Verification items for the finished model (mm, model axes). Round coordinates to 2 decimals unless told otherwise and drop trailing zeros. Order: outer loops, then holes, each group sorted by start corner. A loop starts at its lowest first (then second) coordinate and runs counter-clockwise, first axis right, second up. Notation, with made-up numbers: (-32, 82) -> (-8, 82) arc R21 ccw to (-8, 88) -> close; hole circle Ø4 at (-20, -27.75). An arc over 180 degrees is marked (long way). Put each result on its own line as item: value.
from build123d import *

# Parameters (mm, degrees)
CLAMP_AND_LOWER_FOOT_DEPTH = 14
SKETCH_2_R                 = 57.15
CANISTER_SEAT_DEPTH        = 89.959640287


with BuildPart() as part:
    # 草图1 → Clamp_and_lower_foot (new body)
    with BuildSketch(Plane.XY):
        Polygon((39.852831801, -47.494755473), (43.840620434, -43.840620434), (47.494755473, -39.852831801), (50.787426746, -35.561739054), (53.693575035, -31), (56.191082796, -26.202332228), (58.260942489, -21.205248886), (59.88740123, -16.046780796), (61.058080687, -10.766187015), (61.764071282, -5.40365605), (62, 0), (61.764071282, 5.40365605), (61.058080687, 10.766187015), (59.88740123, 16.046780796), (58.260942489, 21.205248886), (56.191082796, 26.202332228), (53.693575035, 31), (50.787426746, 35.561739054), (47.494755473, 39.852831801), (43.840620434, 43.840620434), (39.852831801, 47.494755473), (35.561739054, 50.787426746), (31, 53.693575035), (26.202332228, 56.191082796), (21.205248886, 58.260942489), (16.046780796, 59.88740123), (10.766187015, 61.058080687), (5.40365605, 61.764071282), (0, 62), (-5.40365605, 61.764071282), (-10.766187015, 61.058080687), (-16.046780796, 59.88740123), (-21.205248886, 58.260942489), (-26.202332228, 56.191082796), (-31, 53.693575035), (-35.561739054, 50.787426746), (-39.852831801, 47.494755473), (-43.840620434, 43.840620434), (-47.494755473, 39.852831801), (-50.787426746, 35.561739054), (-53.693575035, 31), (-56.191082796, 26.202332228), (-58.260942489, 21.205248886), (-59.88740123, 16.046780796), (-61.058080687, 10.766187015), (-61.764071282, 5.40365605), (-62, 0), (-61.764071282, -5.40365605), (-61.058080687, -10.766187015), (-59.88740123, -16.046780796), (-58.260942489, -21.205248886), (-56.191082796, -26.202332228), (-53.693575035, -31), (-50.787426746, -35.561739054), (-47.494755473, -39.852831801), (-43.840620434, -43.840620434), (-39.852831801, -47.494755473), (-0.0065, -62.24), (29.9935, -62.24), align=None)
    extrude(amount=CLAMP_AND_LOWER_FOOT_DEPTH)

    # 草图2 → Canister_seat (cut, through all)
    with BuildSketch(Plane.XY.offset(14)):
        Circle(SKETCH_2_R)
    extrude(amount=-CANISTER_SEAT_DEPTH, mode=Mode.SUBTRACT)


solid = part.part
Item 1: Material ranges on L1, parallel to Y at x = 0, z = 9; L2, parallel to Y at x = 33, z = 7; L3, parallel to X at y = -1, z = 10.5, recorded low to high. Write a range as [from, to].
Check sheet entries:
L1: y = [-62.24, -57.15], [57.15, 62]
L2: y = [-57.74, -46.66], [46.66, 52.42]
L3: x = [-61.96, -57.14], [57.14, 61.96]
Item 2: Gauge pin test, flat ends, axial feed: pin 1 Ø1 at (x, z) = (-27.5, 10.5) entering from +Y; pin 2 Ø5 at (x, z) = (-24.5, 4) entering from +Y; pin 3 Ø8 at (x, z) = (-42.5, 6.5) entering from -Y. Record the tip position at first contact, or that the pin passes through.
Check sheet entries:
pin 1: stops at y = 55.78
pin 2: stops at y = 57.93
pin 3: stops at y = -48
Item 3: Section check A-A on x = -37. Record the boundary of the cut face in (y, z).
Check sheet entries:
outline: (-48.55, 0) -> (-43.56, 0) -> (-43.56, 14) -> (-48.55, 14) -> close; (43.56, 0) -> (49.68, 0) -> (49.68, 14) -> (43.56, 14) -> close
Item 4: Section check B-B on x = -14.5. Record the boundary of the cut face in (y, z), then the cut area to 3 significant figures.
Check sheet entries:
outline: (-56.88, 0) -> (-55.28, 0) -> (-55.28, 14) -> (-56.88, 14) -> close; (55.28, 0) -> (60.23, 0) -> (60.23, 14) -> (55.28, 14) -> close
area: 91.7 mm^2
Item 5: Release check for a two-part mould opening along X. For faces 1 (the cylindrical face through (-57.095, 2.513, 7.098)), 2 (the flat face through (59.063, -18.662, 6.902)), 3 (the flat face through (-49.118, 37.737, 6.902)) record: +X half, -X half, draft (parallel to the pull), parting line (faces both ways), or undercut.
Check sheet entries:
face 1: undercut
face 2: +X half
face 3: -X half
